Check sheet for the modelled part. Datum: model origin and axes. Units: mm. A direction names the side the tool comes from. Round coordinates to 2 decimals unless told otherwise and drop trailing zeros. Write each loop counter-clockwise with the first axis right and the second up, starting at its lowest first coordinate (ties: lowest second). Pieces come first, ordered by that corner, then holes. Notation, with made-up numbers: M 22,73.25 L 63,73.25 A21 cw 63,78.25 Z; hole C -8,12 d11. An arc over 180 degrees is marked long. Answer in a Markdown table with one row per item.
```python
from build123d import *

# Parameters (mm, degrees)
SKETCH1_R               = 14.5
BOSS_EXTRUDE1_DEPTH     = 16
SKETCH2_R               = 11
BOSS_EXTRUDE2_DEPTH     = 12
CUT_EXTRUDE1_DEPTH      = 27.009613607
CUT_EXTRUDE1_DEPTH_BACK = 27.009613607
SKETCH3_R               = 4


with BuildPart() as part:
    # Sketch1 → Boss-Extrude1 (new body)
    with BuildSketch(Plane.XY):
        Circle(SKETCH1_R)
    extrude(amount=BOSS_EXTRUDE1_DEPTH)

    # Sketch2 → Boss-Extrude2 (add)
    with BuildSketch(Plane.XY):
        Circle(SKETCH2_R)
    extrude(amount=-BOSS_EXTRUDE2_DEPTH)

    # Sketch3 → Cut-Extrude1 (cut, two sides: drawn at the far end of the back side and taken through both)
    with BuildSketch(Plane.XY.offset(-CUT_EXTRUDE1_DEPTH_BACK)):
        Circle(SKETCH3_R)
    extrude(amount=CUT_EXTRUDE1_DEPTH + CUT_EXTRUDE1_DEPTH_BACK, mode=Mode.SUBTRACT)


solid = part.part
```
1. Section check D-D, the plane y = 7.75. Record the cut outline in (x, z).
Found:
| item | result |
|---|---|
| outline | M -12.26,0 L -7.81,0 L -7.81,-12 L 7.81,-12 L 7.81,0 L 12.26,0 L 12.26,16 L -12.26,16 Z |
2. Go/stop test with flat-tipped pins: pin 1 (7 mm diameter, centred on x = 0, y = 0, fed in from +Z); pin 2 (1.5 mm diameter, centred on x = 0, z = -6, fed in from -Y); pin 3 (4 mm diameter, centred on y = 6.5, z = 9, fed in from -X). Record where each tip stops, or that it passes through.
Found:
| item | result |
|---|---|
| pin 1 | passes through |
| pin 2 | stops at y = -11 |
| pin 3 | stops at x = -13.78 |
3. Scan lines: L1, parallel to Y at x = 0, z = 6; L2, parallel to X at y = 0.25, z = -7.75; L3, parallel to Y at x = 0, z = -6. Record each from-to range of solid material in increasing order.
Found:
| item | result |
|---|---|
| L1 | y = -14.5 to -4, 4 to 14.5 |
| L2 | x = -11 to -3.99, 3.99 to 11 |
| L3 | y = -11 to -4, 4 to 11 |
4. Section check C-C, the plane z = 11. Record the cut outline in (x, y).
Found:
| item | result |
|---|---|
| outline | C 0,0 d29; hole C 0,0 d8 |
5. Section check A-A, the plane x = 0. Record the cut outline in (y, z), and give its area (3 significant figures).
Found:
| item | result |
|---|---|
| outline | M -14.5,0 L -11,0 L -11,-12 L -4,-12 L -4,16 L -14.5,16 Z; M 4,-12 L 11,-12 L 11,0 L 14.5,0 L 14.5,16 L 4,16 Z |
| area | 504 mm2 |
6. Access from +Z, -Z, +X, -X, +Y, -Y to the whole of each face (thin tool, end or side, straight path). Record for faces 1 (the face through (-2, 11, 0)), 2 (the face through (3, -3, 16)).
Found:
| item | result |
|---|---|
| face 1 | -Z |
| face 2 | +Z, +X, -X, +Y, -Y |
